Build history of the part. All positions in model axes, mm. Face numbers are marked on the shaded views. A direction names the side the tool comes from. Give positions to 0.01 mm unless a question says otherwise; leave off trailing zeros. Write each loop counter-clockwise with the first axis right and the second up, starting at its lowest first coordinate (ties: lowest second). Pieces come first, ordered by that corner, then holes. Notation, with made-up numbers: M -8,-8 L 6,-8 A33 cw 6,23 Z; hole C -35,65.5 d6. An arc over 180 degrees is marked long. One line per item, written item: value. Start each with the question number.
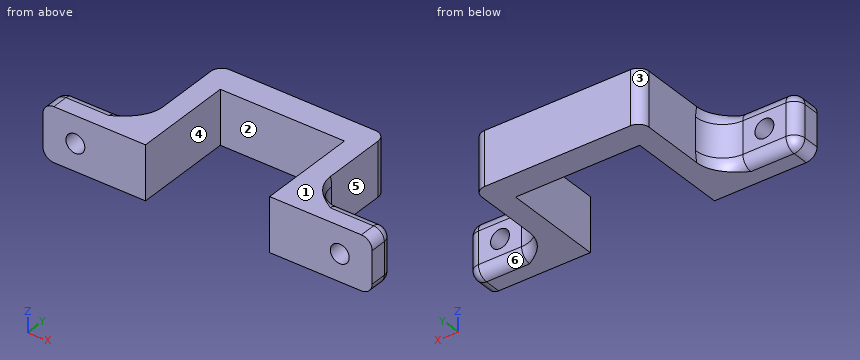
from build123d import *

# Parameters (mm, degrees)
SKETCH1_W           = 15
SKETCH1_H           = 10
SKETCH1_W_2         = 4
SKETCH1_W_3         = 23
BOSS_EXTRUDE1_DEPTH = 23.5
SKETCH1_3_W         = 23
SKETCH1_3_H         = 10
CUT_EXTRUDE1_DEPTH  = 18.5
CUT_EXTRUDE2_START  = 23.5
SKETCH1_4_W         = 15
SKETCH1_4_H         = 10
CUT_EXTRUDE2_DEPTH  = 18.5
FILLET1_R           = 2
FILLET2_R           = 2
FILLET3_R           = 5
CUT_EXTRUDE3_REACH  = 48.971
SKETCH2_R           = 1.75


with BuildPart() as part:
    # Sketch1 → Boss-Extrude1 (new body)
    with BuildSketch(Plane(origin=(0, 0, 0), x_dir=(1, 0, 0), z_dir=(0, 1, 0))):
        with Locations((-34.5, -5)):
            Rectangle(SKETCH1_W, SKETCH1_H)
        with Locations((-25, -5)):
            Rectangle(SKETCH1_W_2, SKETCH1_H)
        with Locations((-11.5, -5)):
            Rectangle(SKETCH1_W_3, SKETCH1_H)
        with Locations((2, -5)):
            Rectangle(SKETCH1_W_2, SKETCH1_H)
        with Locations((11.5, -5)):
            Rectangle(SKETCH1_W, SKETCH1_H)
    extrude(amount=BOSS_EXTRUDE1_DEPTH)

    # Sketch1<3> → Cut-Extrude1 (cut)
    with BuildSketch(Plane(origin=(0, 0, 0), x_dir=(1, 0, 0), z_dir=(0, 1, 0))):
        with Locations((-11.5, -5)):
            Rectangle(SKETCH1_3_W, SKETCH1_3_H)
    extrude(amount=CUT_EXTRUDE1_DEPTH, mode=Mode.SUBTRACT)

    # Sketch1<4> → Cut-Extrude2 (cut)
    with BuildSketch(Plane(origin=(0, 0, 0), x_dir=(1, 0, 0), z_dir=(0, 1, 0)).offset(CUT_EXTRUDE2_START)):
        with Locations((-34.5, -5)):
            Rectangle(SKETCH1_4_W, SKETCH1_4_H)
        with Locations((11.5, -5)):
            Rectangle(SKETCH1_4_W, SKETCH1_4_H)
    extrude(amount=-CUT_EXTRUDE2_DEPTH, mode=Mode.SUBTRACT)

    # Fillet1
    fillet1_edges = [part.edges().sort_by_distance(p)[0] for p in [
        (19, 2.5, 0),
        (19, 2.5, 10),
        (-42, 2.5, 10),
        (-42, 2.5, 0),
        (-27, 23.5, 5),
        (4, 23.5, 5),
    ]]
    fillet(fillet1_edges, radius=FILLET1_R)

    # Fillet2
    fillet2_edges = [part.edges().sort_by_distance(p)[0] for p in [
        (-33.5, 5, 0),
        (-33.5, 5, 10),
        (10.5, 5, 10),
        (10.5, 5, 0),
        (19, 5, 5),
        (18.414213562, 5, 9.414213562),
        (18.414213562, 5, 0.585786438),
        (-42, 5, 5),
        (-41.414213562, 5, 9.414213562),
        (-41.414213562, 5, 0.585786438),
    ]]
    fillet(fillet2_edges, radius=FILLET2_R)

    # Fillet3
    # the kernel refuses this fillet: 5 mm, written as the material it adds along each edge
    with BuildSketch(Plane(origin=(-27, 5, 8), x_dir=(-1, 0, 0), z_dir=(0, 0, -1))) as fillet3_piece_1:
        with BuildLine():
            CenterArc((FILLET3_R, FILLET3_R), FILLET3_R, 180, 90)
            Line((0, FILLET3_R), (0, 0))
            Line((0, 0), (FILLET3_R, 0))
        make_face()
    extrude(amount=6)
    with BuildSketch(Plane(origin=(4, 5, 8), x_dir=(1, 0, 0), z_dir=(0, 0, -1))) as fillet3_piece_2:
        with BuildLine():
            CenterArc((FILLET3_R, -FILLET3_R), FILLET3_R, 90, 90)
            Line((0, -FILLET3_R), (0, 0))
            Line((0, 0), (FILLET3_R, 0))
        make_face()
    extrude(amount=6)
    with BuildSketch(Plane(origin=(-27, 3, 8), x_dir=(0, 0.9999802608561372, -0.006283143965558846), z_dir=(0, 0.006283143965558846, 0.9999802608561372))) as fillet3_piece_3_section:
        with BuildLine():
            CenterArc((-2 - FILLET3_R, FILLET3_R), FILLET3_R, 270, 90)
            Line((-2 - FILLET3_R, 0), (-2, 0))
            Line((-2, 0), (-2, FILLET3_R))
        make_face()
    fillet3_piece_3 = revolve(axis=Axis((-27, 3, 8), (-1, 0, 0)), revolution_arc=359.64, mode=Mode.PRIVATE)
    fillet3_piece_3 = split(fillet3_piece_3, bisect_by=Plane(origin=(-28.84257052, 4.524977571, 10), z_dir=(0, 0, -1)), keep=Keep.TOP, mode=Mode.PRIVATE)
    fillet3_piece_3 = split(fillet3_piece_3, bisect_by=Plane(origin=(-28.84257052, 0, 9.524977571), z_dir=(0, 1, 0)), keep=Keep.TOP, mode=Mode.PRIVATE)
    add(fillet3_piece_3)
    with BuildSketch(Plane(origin=(4, 3, 8), x_dir=(0, 1, 0), z_dir=(0, 0, -1))) as fillet3_piece_4_section:
        with BuildLine():
            CenterArc((2 + FILLET3_R, FILLET3_R), FILLET3_R, 180, 90)
            Line((2 + FILLET3_R, 0), (2, 0))
            Line((2, 0), (2, FILLET3_R))
        make_face()
    fillet3_piece_4 = revolve(axis=Axis((4, 3, 8), (1, 0, 0)), revolution_arc=359.64, mode=Mode.PRIVATE)
    fillet3_piece_4 = split(fillet3_piece_4, bisect_by=Plane(origin=(5.842570594, 4.524977559, 10), z_dir=(0, 0, -1)), keep=Keep.TOP, mode=Mode.PRIVATE)
    fillet3_piece_4 = split(fillet3_piece_4, bisect_by=Plane(origin=(5.842570594, 0, 9.524977563), z_dir=(0, 1, 0)), keep=Keep.TOP, mode=Mode.PRIVATE)
    add(fillet3_piece_4)
    with BuildSketch(Plane(origin=(-27, 3, 2), x_dir=(0, 0.9999802608561372, 0.006283143965559623), z_dir=(0, 0.006283143965559623, -0.9999802608561372))) as fillet3_piece_5_section:
        with BuildLine():
            CenterArc((-2 - FILLET3_R, -FILLET3_R), FILLET3_R, 0, 90)
            Line((-2 - FILLET3_R, 0), (-2, 0))
            Line((-2, 0), (-2, -FILLET3_R))
        make_face()
    fillet3_piece_5 = revolve(axis=Axis((-27, 3, 2), (1, 0, 0)), revolution_arc=359.64, mode=Mode.PRIVATE)
    fillet3_piece_5 = split(fillet3_piece_5, bisect_by=Plane(origin=(-28.842570484, 4.524977653, 0), z_dir=(0, 0, 1)), keep=Keep.TOP, mode=Mode.PRIVATE)
    fillet3_piece_5 = split(fillet3_piece_5, bisect_by=Plane(origin=(-28.842570484, 0, 0.47502245), z_dir=(0, 1, 0)), keep=Keep.TOP, mode=Mode.PRIVATE)
    add(fillet3_piece_5)
    with BuildSketch(Plane(origin=(4, 3, 2), x_dir=(0, 1, 0), z_dir=(0, 0, 1))) as fillet3_piece_6_section:
        with BuildLine():
            CenterArc((2 + FILLET3_R, -FILLET3_R), FILLET3_R, 90, 90)
            Line((2, -FILLET3_R), (2, 0))
            Line((2, 0), (2 + FILLET3_R, 0))
        make_face()
    fillet3_piece_6 = revolve(axis=Axis((4, 3, 2), (-1, 0, 0)), revolution_arc=359.64, mode=Mode.PRIVATE)
    fillet3_piece_6 = split(fillet3_piece_6, bisect_by=Plane(origin=(4.944030812, 6.137069115, 0), z_dir=(0, 0, 1)), keep=Keep.TOP, mode=Mode.PRIVATE)
    fillet3_piece_6 = split(fillet3_piece_6, bisect_by=Plane(origin=(4.944030812, 0, 1.077199574), z_dir=(0, 1, 0)), keep=Keep.TOP, mode=Mode.PRIVATE)
    add(fillet3_piece_6)

    # Sketch2 → Cut-Extrude3 (cut, up to next)
    with BuildSketch(Plane(origin=(0, 5, 0), x_dir=(1, 0, 0), z_dir=(0, 1, 0)), mode=Mode.PRIVATE) as cut_extrude3_sk1:
        with Locations(Location((13, -5, 0), (0, 0, 270))):
            Circle(SKETCH2_R)
    cut_extrude3_tool1 = extrude(cut_extrude3_sk1.sketch, amount=-CUT_EXTRUDE3_REACH, mode=Mode.PRIVATE) & part.part
    # Sketch2 → Cut-Extrude3 (cut, up to next)
    with BuildSketch(Plane(origin=(0, 5, 0), x_dir=(1, 0, 0), z_dir=(0, 1, 0)), mode=Mode.PRIVATE) as cut_extrude3_sk2:
        with Locations(Location((-36, -5, 0), (0, 0, 270))):
            Circle(SKETCH2_R)
    cut_extrude3_tool2 = extrude(cut_extrude3_sk2.sketch, amount=-CUT_EXTRUDE3_REACH, mode=Mode.PRIVATE) & part.part
    add(cut_extrude3_tool1.solids().sort_by_distance((13, 5, 5))[0], mode=Mode.SUBTRACT)
    add(cut_extrude3_tool2.solids().sort_by_distance((-36, 5, 5))[0], mode=Mode.SUBTRACT)


solid = part.part
1) Band-saw the part on D-D (y = 20.5). List the corners of the cut face in (x, z), then the cut area to 3 significant figures.
2) Mould opens along X. For the marked faces 1, 2 and 3 say: released by +X, released by -X, zero draft, split by the parting line, or undercut.
3) Band-saw the part on C-C (y = 14.25). List the corners of the cut face in (x, z), then the cut area to 3 significant figures.
4) Drop flat-ended pins along their axis: P1, Ø2, axis at x = -26, z = 3, coming from the +Y side; P2, Ø2, axis at x = 13, z = 5, coming from the -Y side; P3, Ø5, axis at y = 15.5, z = 4, coming from the +X side; P4, Ø3, axis at x = 11.5, z = 3.5, coming from the +Y side. Give the stop position or say it passes through.
5) Tool access for the marked faces 4, 5 and 6: list every direction of +Z, -Z, +X, -X, +Y, -Y with a clear straight run to the whole face (end or side of a thin tool).
6) Probe line 1 along X through (y, z) = (1.4, 5); line 2 along X through (y, z) = (11, 5.75); line 3 along X through (y, z) = (3.7, 5). List the from-to ranges inside material, lowest first. Write a range as from..to.
7) Band-saw the part on A-A (x = 13). List the corners of the cut face in (y, z), then the cut area to 3 significant figures.
8) Band-saw the part on B-B (z = 5). List the corners of the cut face in (x, y).
Model answer:
1. outline: M -27,0 L 4,0 L 4,10 L -27,10 Z
1. area: 310 mm²
2. face 1: zero draft
2. face 2: undercut
2. face 3: released by -X
3. outline: M -27,0 L -23,0 L -23,10 L -27,10 Z; M 0,0 L 4,0 L 4,10 L 0,10 Z
3. area: 80.0 mm²
4. P1: stops at y = 23.5
4. P2: passes through
4. P3: stops at x = 4
4. P4: stops at y = 5
5. face 4: +Z, -Z, -Y
5. face 5: +Z, -Z, +X, +Y
5. face 6: -Z, +X, +Y
6. line 1: x = -42..-37.75, -34.25..-23, 0..11.25, 14.75..19
6. line 2: x = -27..-23, 0..4
6. line 3: x = -41.87..-37.75, -34.25..-23, 0..11.25, 14.75..18.87
7. outline: M 0,0 L 3,0 A2 ccw 5,2 L 5,3.25 L 0,3.25 Z; M 0,6.75 L 5,6.75 L 5,8 A2 ccw 3,10 L 0,10 Z
7. area: 30.8 mm²
8. outline: M -42,0 L -37.75,0 L -37.75,5 L -40,5 A2 ccw -42,3 Z; M -34.25,0 L -23,0 L -23,18.5 L 0,18.5 L 0,0 L 11.25,0 L 11.25,5 L 9,5 A5 cw 4,10 L 4,21.5 A2 ccw 2,23.5 L -25,23.5 A2 ccw -27,21.5 L -27,10 A5 cw -32,5 L -34.25,5 Z; M 14.75,0 L 19,0 L 19,3 A2 ccw 17,5 L 14.75,5 Z
